Print and shaded views of the part. All mm, measured from the part's lowest x, y and z. Give positions to 0.01 mm unless a question says otherwise; leave off trailing zeros. Loops run counter-clockwise (first coordinate to the right, second up) from the corner with the lowest first, then second, coordinate; pieces in that order, holes last.
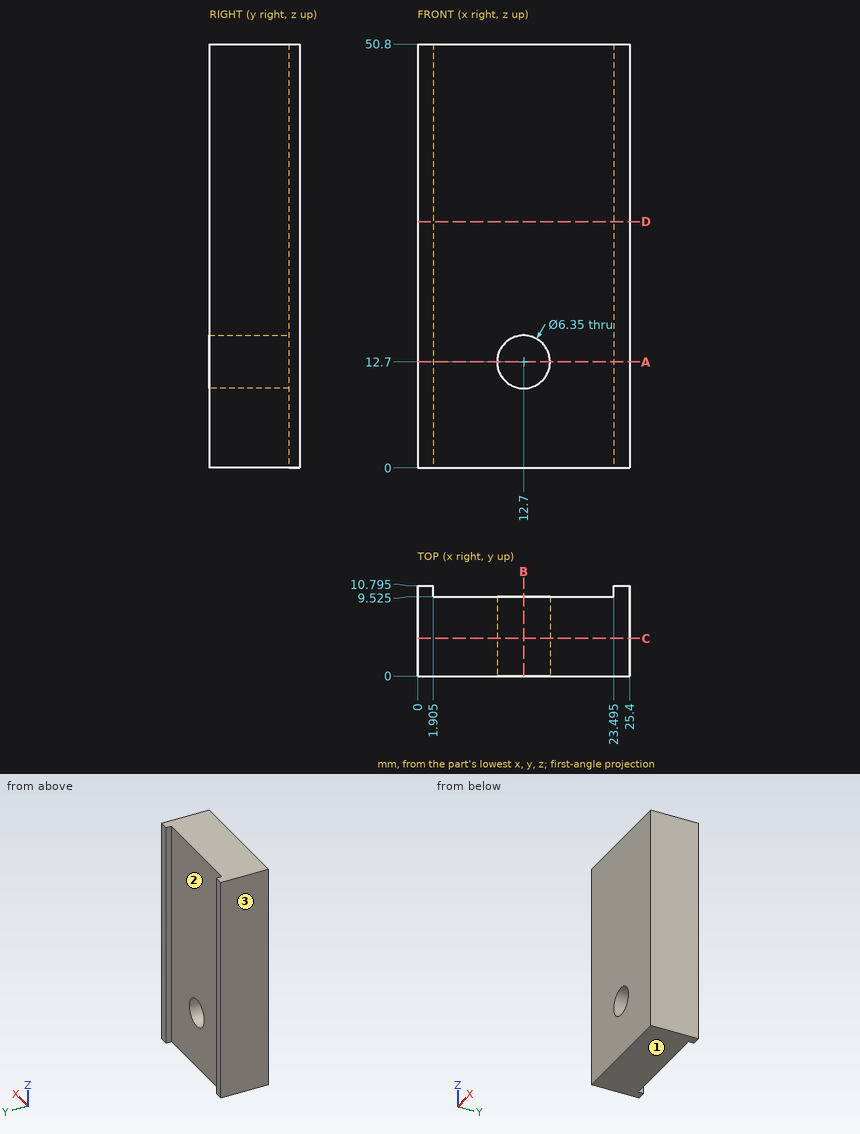
1. Saw through at D-D, the plane z = 29.5. List the corners of the cut face in (x, y) (3 decimals).
Responses:
outline: (0, 0) - (25.4, 0) - (25.4, 10.795) - (23.495, 10.795) - (23.495, 9.525) - (1.905, 9.525) - (1.905, 10.795) - (0, 10.795) - close
2. Drop a flat-ended pin along its axis: pin 1 (6 mm diameter, centred on x = 12.5, z = 36.5, fed in from +Y) (3 decimals). Give the stop position or say it passes through.
Responses:
pin 1: stops at y = 9.525
3. Probe line 1 along X through (y, z) = (7.75, 12.7) (3 decimals); line 2 along Y through (x, z) = (9.5, 42.5) (3 decimals); line 3 along X through (y, z) = (9.75, 19) (3 decimals). List the from-to ranges inside material, lowest first.
Responses:
line 1: x = 0 to 9.525, 15.875 to 25.4
line 2: y = 0 to 9.525
line 3: x = 0 to 1.905, 23.495 to 25.4
4. Saw through at C-C, the plane y = 4.5. List the corners of the cut face in (x, z) (3 decimals).
Responses:
outline: (0, 0) - (25.4, 0) - (25.4, 50.8) - (0, 50.8) - close; hole circle Ø6.35 at (12.7, 12.7)
5. Saw through at A-A, the plane z = 12.7. List the corners of the cut face in (x, y) (3 decimals), and give its area (3 significant figures).
Responses:
outline: (0, 0) - (9.525, 0) - (9.525, 9.525) - (1.905, 9.525) - (1.905, 10.795) - (0, 10.795) - close; (15.875, 0) - (25.4, 0) - (25.4, 10.795) - (23.495, 10.795) - (23.495, 9.525) - (15.875, 9.525) - close
area: 186 mm2
6. Pull direction X, two halves, no side cores. Call the marked faces 1, 2 and 3: released by +X, released by -X, zero draft, split by the parting line, or undercut.
Responses:
face 1: zero draft
face 2: undercut
face 3: released by -X
7. Saw through at B-B, the plane x = 12.7. List the corners of the cut face in (y, z) (3 decimals).
Responses:
outline: (0, 0) - (9.525, 0) - (9.525, 9.525) - (0, 9.525) - close; (0, 15.875) - (9.525, 15.875) - (9.525, 50.8) - (0, 50.8) - close
